```python
from build123d import *

# Parameters (mm, degrees)
BOSS_EXTRU_1_DEPTH      = 6
ESQUISSE2_R             = 1.5
ENL_V_MAT_EXTRU_1_DEPTH = 5
ESQUISSE3_R             = 0.625
ENL_V_MAT_EXTRU_2_DEPTH = 35.058772732
CONG_2_R                = 1
CONG_3_R                = 1


with BuildPart() as part:
    # Esquisse1 → Boss.-Extru.1 (new body)
    with BuildSketch(Plane.XY):
        Polygon((-12, 10), (-16, 10), (-16, -10), (16, -10), (16, 10), (12, 10), (12, -5), (-12, -5), align=None)
    extrude(amount=BOSS_EXTRU_1_DEPTH)

    # Esquisse2 → Enlèv. mat.-Extru.1 (cut)
    with BuildSketch(Plane(origin=(0, -5, 0), x_dir=(1, 0, 0), z_dir=(0, 1, 0))):
        with Locations(Location((0, -3, 0), (0, 0, 270))):
            Circle(ESQUISSE2_R)
    extrude(amount=-ENL_V_MAT_EXTRU_1_DEPTH, mode=Mode.SUBTRACT)

    # Esquisse3 → Enlèv. mat.-Extru.2 (cut, through all)
    with BuildSketch(Plane(origin=(16, 0, 0), x_dir=(0, 0, -1), z_dir=(1, 0, 0))):
        with Locations((-3.5, 5)):
            Circle(ESQUISSE3_R)
        with Locations((-3.5, -2)):
            Circle(ESQUISSE3_R)
    extrude(amount=-ENL_V_MAT_EXTRU_2_DEPTH, mode=Mode.SUBTRACT)

    # Congé2
    cong_2_edges = [part.edges().sort_by_distance(p)[0] for p in [
        (-12, -5, 3),
    ]]
    fillet(cong_2_edges, radius=CONG_2_R)

    # Congé3
    cong_3_edges = [part.edges().sort_by_distance(p)[0] for p in [
        (12, -5, 3),
    ]]
    fillet(cong_3_edges, radius=CONG_3_R)


solid = part.part
```
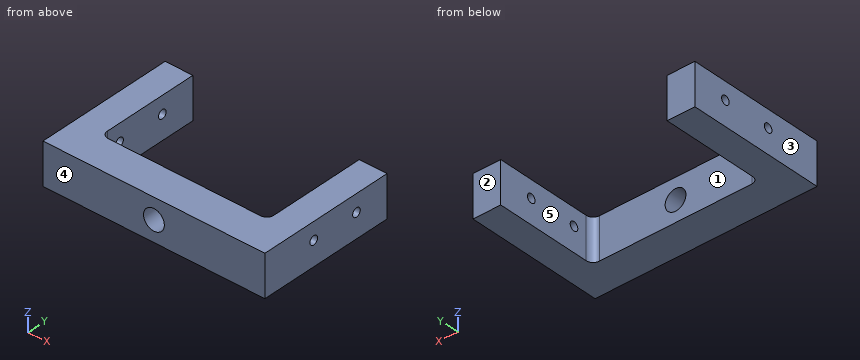
Read the model definition and answer for the solid it produces. Units are mm, in the model's axes. Face numbers are marked on the shaded views. A direction names the side the tool comes from. Round coordinates to 2 decimals unless told otherwise and drop trailing zeros. Write each loop counter-clockwise with the first axis right and the second up, starting at its lowest first coordinate (ties: lowest second). Pieces come first, ordered by that corner, then holes. Notation, with made-up numbers: (-5.5, -23) -> (45.5, -23) arc R18 ccw to (45.5, -18) -> close; hole circle Ø1 at (-16, -39.5). An arc over 180 degrees is marked (long way). Answer in a Markdown table with one row per item. Add a question column.
1) Find section C-C, the plane y = -2. Determine the outline of the cut face in (x, z) (3 decimals), and give its area (3 significant figures).
2) Which of the six approach directions +Z, -Z, +X, -X, +Y, -Y give full straight-line access (tool end or side, diameter ignored) to the marked faces 4 and 5?
3) Find section D-D, the plane z = 3.5. State how many separate pieces and enclosed holes the cut face has, and give its area (3 significant figures).
4) Find section B-B, the plane y = 1. Determine the outline of the cut face in (x, z), and give its area (3 significant figures).
5) Given P1, Ø2, axis at x = -1, z = 5, coming from the +Y side, flat-ended and moving along its own axis, determine where the tip first touches the part or whether it passes through.
6) Consider line 1 (Y direction, x = -14.7, z = 3.5) (3 decimals); line 2 (X direction, y = -8.55, z = 3); line 3 (X direction, y = 8, z = 2.4). Determine where each line is inside the solid, lowest interval first.
7) Determine the mould class of the marked faces 1, 2 and 3 for opening direction X: pulls with the +X half, pulls with the -X half, needs draft (parallel to the pull), parting line crosses it, or undercut.
8) Find section A-A, the plane x = 0. Determine the outline of the cut face in (y, z).
Findings below:
| question | item | result |
|---|---|---|
| 1 | outline | (-16, 0) -> (-12, 0) -> (-12, 2.875) -> (-16, 2.875) -> close; (-16, 4.125) -> (-12, 4.125) -> (-12, 6) -> (-16, 6) -> close; (12, 0) -> (16, 0) -> (16, 2.875) -> (12, 2.875) -> close; (12, 4.125) -> (16, 4.125) -> (16, 6) -> (12, 6) -> close |
| 1 | area | 38.0 mm² |
| 2 | face 4 | +Z, -Z, +X, -X, -Y |
| 2 | face 5 | +Z, -Z, +Y |
| 3 | separate pieces | 6 |
| 3 | enclosed holes | 0 |
| 3 | area | 246 mm² |
| 4 | outline | (-16, 0) -> (-12, 0) -> (-12, 6) -> (-16, 6) -> close; (12, 0) -> (16, 0) -> (16, 6) -> (12, 6) -> close |
| 4 | area | 48.0 mm² |
| 5 | P1 | y = -5 |
| 6 | line 1 | -10 to -2.625, -1.375 to 4.375, 5.625 to 10 |
| 6 | line 2 | -16 to -1.5, 1.5 to 16 |
| 6 | line 3 | -16 to -12, 12 to 16 |
| 7 | face 1 | undercut |
| 7 | face 2 | needs draft |
| 7 | face 3 | pulls with the -X half |
| 8 | outline | (-10, 0) -> (-5, 0) -> (-5, 1.5) -> (-10, 1.5) -> close; (-10, 4.5) -> (-5, 4.5) -> (-5, 6) -> (-10, 6) -> close |
